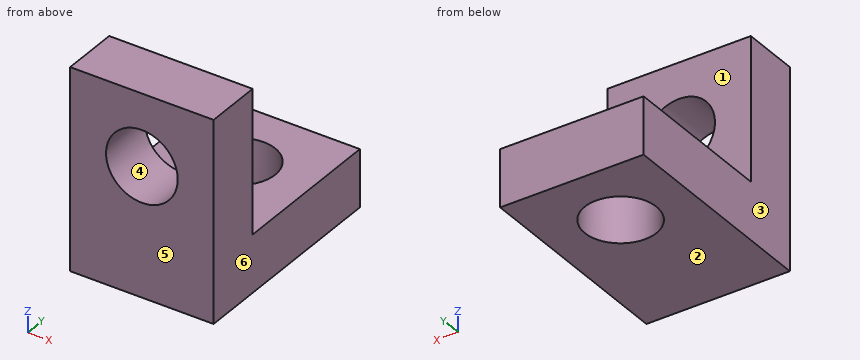
```python
from build123d import *

# Parameters (mm, degrees)
SKETCH1_W           = 10
SKETCH1_H           = 15
SKETCH1_R           = 2.5
BOSS_EXTRUDE1_DEPTH = 4
SKETCH2_W           = 10
SKETCH2_H           = 4
BOSS_EXTRUDE2_DEPTH = 10
SKETCH3_R           = 2.5
CUT_EXTRUDE1_DEPTH  = 10


with BuildPart() as part:
    # Sketch1 → Boss-Extrude1 (new body)
    with BuildSketch(Plane.XY):
        Rectangle(SKETCH1_W, SKETCH1_H)
        with Locations((0, 2.5)):
            Circle(SKETCH1_R, mode=Mode.SUBTRACT)
    extrude(amount=BOSS_EXTRUDE1_DEPTH)

    # Sketch2 → Boss-Extrude2 (add)
    with BuildSketch(Plane.XY.offset(4)):
        with Locations((0, -5.5)):
            Rectangle(SKETCH2_W, SKETCH2_H)
    extrude(amount=BOSS_EXTRUDE2_DEPTH)

    # Sketch3 → Cut-Extrude1 (cut)
    with BuildSketch(Plane(origin=(0, -3.5, 0), x_dir=(1, 0, 0), z_dir=(0, 1, 0))):
        with Locations(Location((0, -9, 0), (0, 0, 270))):
            Circle(SKETCH3_R)
    extrude(amount=-CUT_EXTRUDE1_DEPTH, mode=Mode.SUBTRACT)


solid = part.part
```
CAD build for the part. Positions are in the model's coordinates, mm. Face numbers are marked on the shaded views. A direction names the side the tool comes from. Give positions to 0.01 mm unless a question says otherwise; leave off trailing zeros. Order: outer loops, then holes, each group sorted by start corner. A loop starts at its lowest first (then second) coordinate and runs counter-clockwise, first axis right, second up. Notation, with made-up numbers: M -35.75,-37 L -16.75,-37 A22 cw -16.75,-23 Z; hole C -23,22 d3. An arc over 180 degrees is marked long. Put each result on its own line as item: value. Start each with the question number.
(1) Saw through at B-B, the plane x = 0. Write the cut outline in (y, z).
(2) Saw through at A-A, the plane y = 0.5. Write the cut outline in (x, z).
(3) Saw through at C-C, the plane z = 9. Write the cut outline in (x, y), then the cut area to 3 significant figures.
(4) Mould opens along X. For the marked faces 3, 4, 5 and 6 say: +X half, -X half, draft (parallel to the pull), parting line (faces both ways), or undercut.
(5) Saw through at D-D, the plane y = -3.75. Write the cut outline in (x, z).
(6) Which spindle directions (+Z, -Z, +X, -X, +Y, -Y) get a long thin tool onto all of the face, cutting with end or side? Do the marked faces 1 and 2. Say none if no direction does.
(7) Drill centre lines: line 1 along X through (y, z) = (-4.6, 9); line 2 along Y through (x, z) = (0.5, 11.75); line 3 along Z through (x, y) = (0.25, -4.25). Where is each one in solid material? Low to high.
Check result:
1. outline: M -7.5,0 L 0,0 L 0,4 L -3.5,4 L -3.5,6.5 L -7.5,6.5 Z; M -7.5,11.5 L -3.5,11.5 L -3.5,14 L -7.5,14 Z; M 5,0 L 7.5,0 L 7.5,4 L 5,4 Z
2. outline: M -5,0 L -1.5,0 L -1.5,4 L -5,4 Z; M 1.5,0 L 5,0 L 5,4 L 1.5,4 Z
3. outline: M -5,-7.5 L -2.5,-7.5 L -2.5,-3.5 L -5,-3.5 Z; M 2.5,-7.5 L 5,-7.5 L 5,-3.5 L 2.5,-3.5 Z
3. area: 20.0 mm2
4. face 3: -X half
4. face 4: undercut
4. face 5: draft
4. face 6: +X half
5. outline: M -5,0 L 5,0 L 5,14 L -5,14 Z; hole C 0,9 d5
6. face 1: +Z, +X, -X, +Y
6. face 2: -Z, +X, -X, +Y, -Y
7. line 1: x = -5 to -2.5, 2.5 to 5
7. line 2: y = -7.5 to -3.5
7. line 3: z = 0 to 6.51, 11.49 to 14
